```python
from build123d import *

# Parameters (mm, degrees)
EXTRUDE_1_DEPTH     = 30
FILLET_1_R          = 10
FILLET_2_R          = 10
SKETCH_4_R          = 1.5
CUT_EXTRUDE_1_DEPTH = 4
CUT_EXTRUDE_2_DEPTH = 71.641899783
CUT_EXTRUDE_START   = -4
SKETCH_6_R          = 1.5
CUT_EXTRUDE_3_DEPTH = 4
SKETCH_7_R          = 2.5
CUT_EXTRUDE_4_DEPTH = 0.5


with BuildPart() as part:
    # 草图2 → 凸台-拉伸1 (new body)
    with BuildSketch(Plane(origin=(0, 0, 0), x_dir=(1, 0, 0), z_dir=(0, 1, 0))):
        Polygon((23.688888889, -16.857777778), (23.688888889, 18.142222222), (-28.311111111, 18.142222222), (-28.311111111, -16.857777778), (-32.311111111, -16.857777778), (-32.311111111, 22.142222222), (27.688888889, 22.142222222), (27.688888889, -16.857777778), align=None)
    extrude(amount=EXTRUDE_1_DEPTH)

    # 圆角1
    fillet_1_edges = [part.edges().sort_by_distance(p)[0] for p in [
        (23.688888889, 15, -18.142222222),
        (27.688888889, 15, -22.142222222),
    ]]
    fillet(fillet_1_edges, radius=FILLET_1_R)

    # 圆角2
    fillet_2_edges = [part.edges().sort_by_distance(p)[0] for p in [
        (-28.311111111, 15, -18.142222222),
        (-32.311111111, 15, -22.142222222),
    ]]
    fillet(fillet_2_edges, radius=FILLET_2_R)

    # 草图4 → 切除-拉伸1 (cut)
    with BuildSketch(Plane.ZY.offset(32.311111111)):
        with Locations((-3.006286177, 14.956055529)):
            Circle(SKETCH_4_R)
        with Locations((11.493713823, 14.954055529)):
            Circle(SKETCH_4_R)
        with Locations((4.244713823, 22.205055529)):
            Circle(SKETCH_4_R)
        with Locations((4.242713823, 7.705055529)):
            Circle(SKETCH_4_R)
        with Locations((4.244713823, 14.955055529)):
            Circle(SKETCH_4_R)
    extrude(amount=-CUT_EXTRUDE_1_DEPTH, mode=Mode.SUBTRACT)

    # 草图5 → 切除-拉伸2 (cut, through all)
    with BuildSketch(Plane.ZY.offset(32.311111111)):
        with BuildLine():
            Line((16.857777778, 0), (4.244713823, 0))
            Line((4.244713823, 0), (-12.142222222, 0))
            Line((-12.142222222, 0), (4.244713823, 4.955055529))
            ThreePointArc((4.244713823, 4.955055529), (14.244713823, 14.955055529), (4.244713823, 24.955055529))
            Line((4.244713823, 24.955055529), (-12.142222222, 30))
            Line((-12.142222222, 30), (4.244713823, 30))
            Line((4.244713823, 30), (16.857777778, 30))
            Line((16.857777778, 30), (16.857777778, 0))
        make_face()
    extrude(amount=-CUT_EXTRUDE_2_DEPTH, mode=Mode.SUBTRACT)

    # 草图6 → 切除-拉伸3 (cut)
    with BuildSketch(Plane(origin=(27.688888889, 0, 0), x_dir=(0, 0, -1), z_dir=(1, 0, 0)).offset(CUT_EXTRUDE_START)):
        with Locations(Location((-4.244713823, 14.955055529, 0), (0, 0, 180))):
            Circle(SKETCH_6_R)
    extrude(amount=CUT_EXTRUDE_3_DEPTH, mode=Mode.SUBTRACT)

    # 草图7 → 切除-拉伸4 (cut)
    with BuildSketch(Plane(origin=(27.688888889, 0, 0), x_dir=(0, 0, -1), z_dir=(1, 0, 0))):
        with Locations((-4.244713823, 14.955055529)):
            Circle(SKETCH_7_R)
    extrude(amount=-CUT_EXTRUDE_4_DEPTH, mode=Mode.SUBTRACT)


solid = part.part
```
CAD build for the part. Positions are in the model's coordinates, mm. A direction names the side the tool comes from. Coordinates: 2 decimals unless noted, no trailing zeros. Order: outer loops, then holes, each group sorted by start corner. A loop starts at its lowest first (then second) coordinate and runs counter-clockwise, first axis right, second up. Notation, with made-up numbers: M -28,81 L 24,81 A15 cw 24,97 Z; hole C 23.25,87 d1. An arc over 180 degrees is marked long. Write each question's results on one line, items separated by ' | '. Start each with the question number.
Q1. Cut at B-B (y = 23). List the corners of the cut face in (x, z).
Q2. Cut at D-D (y = 19.5). List the corners of the cut face in (x, z).
Q3. Drill centre lines: probe 1 along X at (y, z) = (7, -6.5); probe 2 along Z at (x, y) = (-10, 12); probe 3 along X at (y, z) = (26, -16). Where is each one in solid material? Low to high. Write a range as from..to.
Q4. Flat gauge pins, fed straight in: P1, Ø1, axis at y = 19, z = -14.5, coming from the +X side; P2, Ø1.5, axis at y = 14, z = 5.5, coming from the +X side; P3, Ø2.5, axis at y = 22.21, z = 4.24, coming from the -X side. Where does each tip first touch, or does it go through?
Q5. Pull direction Y, two halves, no side cores. Call faces 4 (the cylindrical face through (20.837, 15.21, -15.135)), 5 (the cylindrical face through (27.442, 17.063, 2.901)), 6 (the flat face through (25.77, 27.44, -3.83)), 7 (the cylindrical face through (25.414, 13.468, 4.049)): +Y half, -Y half, draft (parallel to the pull), parting line (faces both ways), or undercut.
Q6. Cut at A-A (z = 9). List the corners of the cut face in (x, y).
Q7. Cut at C-C (z = 5). List the corners of the cut face in (x, y), then the cut area to 3 significant figures.
Q8. Which spindle directions (+Z, -Z, +X, -X, +Y, -Y) get a long thin tool onto all of the face, cutting with end or side? Do faces 1 (the flat face through (-1.9, 30, -18.3)), 2 (the cylindrical face through (-30.34, 6.24, 3.92)), 3 (the flat face through (-2, 15, -18.142)). Say none if no direction does.
Found:
1) outline: M -32.31,-12.14 A10 ccw -22.31,-22.14 L 17.69,-22.14 A10 ccw 27.69,-12.14 L 27.69,10.18 L 23.69,10.18 L 23.69,-8.14 A10 cw 13.69,-18.14 L -18.31,-18.14 A10 cw -28.31,-8.14 L -28.31,2.97 L -32.31,2.97 Z; M -32.31,5.52 L -28.31,5.52 L -28.31,10.18 L -32.31,10.18 Z
2) outline: M -32.31,-12.14 A10 ccw -22.31,-22.14 L 17.69,-22.14 A10 ccw 27.69,-12.14 L 27.69,13.15 L 23.69,13.15 L 23.69,-8.14 A10 cw 13.69,-18.14 L -18.31,-18.14 A10 cw -28.31,-8.14 L -28.31,13.15 L -32.31,13.15 Z
3) probe 1: -32.31..-28.31, 23.69..27.69 | probe 2: -22.14..-18.14 | probe 3: -31.54..-24.5, 19.87..26.91
4) P1: x = 27.51 | P2: x = 27.19 | P3: x = 23.69
5) face 4: draft | face 5: undercut | face 6: +Y half | face 7: undercut
6) outline: M -32.31,6.16 L -28.31,6.16 L -28.31,23.75 L -32.31,23.75 Z; M 23.69,6.16 L 27.69,6.16 L 27.69,23.75 L 23.69,23.75 Z
7) outline: M -32.31,4.98 L -28.31,4.98 L -28.31,6.41 L -32.31,6.41 Z; M -32.31,9 L -28.31,9 L -28.31,13.66 L -32.31,13.66 Z; M -32.31,16.25 L -28.31,16.25 L -28.31,20.91 L -32.31,20.91 Z; M -32.31,23.5 L -28.31,23.5 L -28.31,24.93 L -32.31,24.93 Z; M 23.69,4.98 L 27.69,4.98 L 27.69,12.57 L 27.19,12.57 L 27.19,13.66 L 23.69,13.66 Z; M 23.69,16.25 L 27.19,16.25 L 27.19,17.34 L 27.69,17.34 L 27.69,24.93 L 23.69,24.93 Z | area: 117 mm²
8) face 1: +Z, -Z, +X, -X, +Y | face 2: -X | face 3: +Z, +Y, -Y
